For this review, take the finished solid that the model builds, in its own axes (mm). Face numbers are marked on the shaded views. A direction names the side the tool comes from. Round coordinates to 2 decimals unless told otherwise and drop trailing zeros. Order: outer loops, then holes, each group sorted by start corner. A loop starts at its lowest first (then second) coordinate and runs counter-clockwise, first axis right, second up. Notation, with made-up numbers: M 30.5,75 L 58.5,75 A16 cw 58.5,104 Z; hole C 64.5,63.25 d11. An arc over 180 degrees is marked long. Use a Markdown table: item, result.
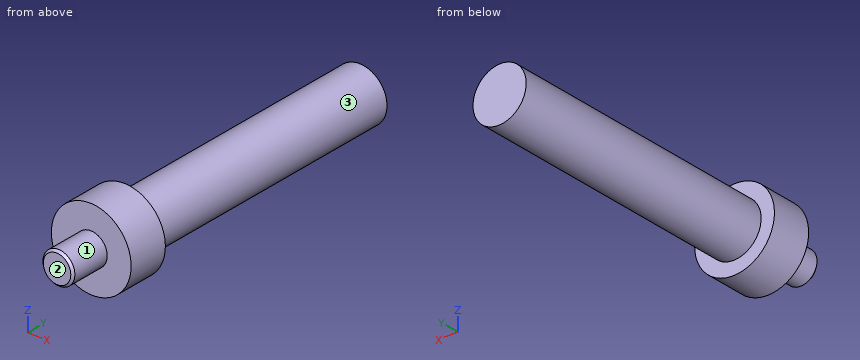
from build123d import *

# Parameters (mm, degrees)
SKETCH1_R           = 15
BOSS_EXTRUDE1_DEPTH = 15
SKETCH2_R           = 10
BOSS_EXTRUDE2_DEPTH = 103
SKETCH3_R           = 7.5
BOSS_EXTRUDE3_DEPTH = 15


# Read off the part's stored shape, not the designer's step: M12x1.5 Machine Threads Stud1
with BuildPart() as part:
    # Sketch1 → Boss-Extrude1 (new body)
    with BuildSketch(Plane(origin=(0, 0, 0), x_dir=(1, 0, 0), z_dir=(0, 1, 0))):
        with Locations(Location((0, 0, 0), (0, 0, 270))):
            Circle(SKETCH1_R)
    extrude(amount=BOSS_EXTRUDE1_DEPTH)

    # Sketch2 → Boss-Extrude2 (add)
    with BuildSketch(Plane(origin=(0, 15, 0), x_dir=(1, 0, 0), z_dir=(0, 1, 0))):
        with Locations(Location((0, 0, 0), (0, 0, 270))):
            Circle(SKETCH2_R)
    extrude(amount=BOSS_EXTRUDE2_DEPTH)

    # Sketch3 → Boss-Extrude3 (add)
    with BuildSketch(Plane.XZ):
        with Locations(Location((0, 0, 0), (0, 0, 270))):
            Circle(SKETCH3_R)
    extrude(amount=BOSS_EXTRUDE3_DEPTH)

    # M12x1.5 Machine Threads Stud1 outline → M12x1.5 Machine Threads Stud1 (revolve, cut)
    with BuildSketch(Plane.XY):
        Polygon((7.5, 0), (6, 0), (6, -14.172), (5.172, -15), (7.5, -15), align=None)
    revolve(axis=Axis((0, 0, 0), (0, 1, 0)), mode=Mode.SUBTRACT)


solid = part.part
Q1. Add section B-B (y = -7). Write out the cut boundary in (x, z), then the cut area to 3 significant figures.
Determined:
| item | result |
|---|---|
| outline | C 0,0 d12 |
| area | 113 mm^2 |
Q2. Add section D-D (y = 95). Write out the cut boundary in (x, z).
Determined:
| item | result |
|---|---|
| outline | C 0,0 d20 |
Q3. Wall thickness on line 1 along Y through (x, z) = (9.5, 4.5); line 2 along Y through (x, z) = (-6.5, 1.25); line 3 along X through (y, z) = (49.5, 9): over which ranges is each line inside the solid? List them lowest first. Write a range as [from, to].
Determined:
| item | result |
|---|---|
| line 1 | y = [0, 15] |
| line 2 | y = [0, 118] |
| line 3 | x = [-4.36, 4.36] |
Q4. Add section C-C (x = 12.75). Write out the cut boundary in (y, z).
Determined:
| item | result |
|---|---|
| outline | M 0,-7.9 L 15,-7.9 L 15,7.9 L 0,7.9 Z |
Q5. Clearance check with flat-ended pins moving along their axes: pin 1 (8 mm diameter, centred on y = 87.5, z = -7, fed in from -X); pin 2 (10 mm diameter, centred on x = 8.5, z = -6, fed in from +Y); pin 3 (12 mm diameter, centred on x = -7.5, z = -11, fed in from -Y); pin 4 (8 mm diameter, centred on x = -8, y = 71.5, fed in from -Z). State where each tip first meets the part, or that it passes through.
Determined:
| item | result |
|---|---|
| pin 1 | stops at x = -9.54 |
| pin 2 | stops at y = 118 |
| pin 3 | stops at y = 0 |
| pin 4 | stops at z = -9.17 |
Q6. Machinability: for the marked faces 1, 2 and 3, which of the approach directions +Z, -Z, +X, -X, +Y, -Y give a long, thin tool a straight path to every point of the face, cutting with its end or side? Answer none if there is none.
Determined:
| item | result |
|---|---|
| face 1 | -Y |
| face 2 | +Z, -Z, +X, -X, -Y |
| face 3 | +Y |
Q7. Add section A-A (z = 0). Write out the cut boundary in (x, y).
Determined:
| item | result |
|---|---|
| outline | M -15,0 L -6,0 L -6,-14.17 L -5.17,-15 L 5.17,-15 L 6,-14.17 L 6,0 L 15,0 L 15,15 L 10,15 L 10,118 L -10,118 L -10,15 L -15,15 Z |
